```python
from build123d import *

# Parameters (mm, degrees)
IZIM1_R                     = 1.65
Y_KSEKLIK_EKSTR_ZYON1_DEPTH = 2.5
RADYUS1_RADIUS              = 3.5
RADYUS1_LENGTH              = 2.5
RADYUS3_R                   = 2
RADYUS4_R                   = 1.5
KES_EKSTR_ZYON1_DEPTH       = 52.79285665


with BuildPart() as part:
    # Çizim1 → Yükseklik-Ekstrüzyon1 (new body)
    with BuildSketch(Plane(origin=(0, 0, 0), x_dir=(0, 0, -1), z_dir=(1, 0, 0))):
        with BuildLine():
            Line((0, 0), (0, 26.5))
            ThreePointArc((0, 26.5), (-0.439339828, 27.560660172), (-1.5, 28))
            Line((-1.5, 28), (-35, 28))
            Line((-35, 28), (-35, 7))
            Line((-35, 7), (-43.5, 7))
            Line((-43.5, 7), (-43.5, 0))
            Line((-43.5, 0), (0, 0))
        make_face()
        with Locations((-17.5, 23.3)):
            Circle(IZIM1_R, mode=Mode.SUBTRACT)
        with Locations((-17.5, 4.7)):
            Circle(IZIM1_R, mode=Mode.SUBTRACT)
        with Locations((-30.9, 6.2)):
            Circle(IZIM1_R, mode=Mode.SUBTRACT)
        with Locations((-30.9, 21.8)):
            Circle(IZIM1_R, mode=Mode.SUBTRACT)
        with Locations((-4.1, 6.2)):
            Circle(IZIM1_R, mode=Mode.SUBTRACT)
        with Locations((-4.1, 21.8)):
            Circle(IZIM1_R, mode=Mode.SUBTRACT)
        with Locations((-40, 3.5)):
            Circle(IZIM1_R, mode=Mode.SUBTRACT)
    extrude(amount=Y_KSEKLIK_EKSTR_ZYON1_DEPTH)

    # Radyus1: full round fillet: the end face becomes a half cylinder, R = half its width
    radyus1_face = Plane((1.25, 3.5, 43.5), x_dir=(1, 0, 0), z_dir=(0, 0, 1))  # on the end face: x along it, z out of the body
    radyus1_slab = radyus1_face.offset(-RADYUS1_RADIUS / 2) * Box(RADYUS1_LENGTH, 2 * RADYUS1_RADIUS, RADYUS1_RADIUS, mode=Mode.PRIVATE)  # the body's end, R deep
    radyus1_round = Plane((1.25, 3.5, 40), x_dir=(0, 0, 1), z_dir=(1, 0, 0)) * Cylinder(RADYUS1_RADIUS, RADYUS1_LENGTH, mode=Mode.PRIVATE)  # its axis R under the face
    add(radyus1_slab - radyus1_round, mode=Mode.SUBTRACT)

    # Radyus3
    radyus3_edges = [part.edges().sort_by_distance(p)[0] for p in [
        (1.25, 7, 35),
    ]]
    fillet(radyus3_edges, radius=RADYUS3_R)

    # Radyus4
    radyus4_edges = [part.edges().sort_by_distance(p)[0] for p in [
        (1.25, 28, 35),
    ]]
    fillet(radyus4_edges, radius=RADYUS4_R)

    # Çizim2 → Kes-Ekstrüzyon1 (cut, through all)
    with BuildSketch(Plane(origin=(2.5, 0, 0), x_dir=(0, 0, -1), z_dir=(1, 0, 0))):
        with BuildLine():
            Line((-33.5, 16.8), (-33.5, 11.8))
            ThreePointArc((-33.5, 11.8), (-33.060660172, 10.739339828), (-32, 10.3))
            Line((-32, 10.3), (-28, 10.3))
            ThreePointArc((-28, 10.3), (-26.648045146, 11.150216904), (-26.828696786, 12.737042571))
            Line((-26.828696786, 12.737042571), (-30.828696786, 17.737042571))
            ThreePointArc((-30.828696786, 17.737042571), (-32.496510412, 18.215442479), (-33.5, 16.8))
        make_face()
        with BuildLine():
            Line((-25, 18.3), (-21, 18.3))
            ThreePointArc((-21, 18.3), (-19.939339828, 17.860660172), (-19.5, 16.8))
            Line((-19.5, 16.8), (-19.5, 11.8))
            ThreePointArc((-19.5, 11.8), (-20.503489588, 10.384557521), (-22.171303214, 10.862957429))
            Line((-22.171303214, 10.862957429), (-26.171303214, 15.862957429))
            ThreePointArc((-26.171303214, 15.862957429), (-26.351954854, 17.449783096), (-25, 18.3))
        make_face()
        with BuildLine():
            Line((-12.828696786, 10.862957429), (-8.828696786, 15.862957429))
            ThreePointArc((-8.828696786, 15.862957429), (-8.648045146, 17.449783096), (-10, 18.3))
            Line((-10, 18.3), (-14, 18.3))
            ThreePointArc((-14, 18.3), (-15.060660172, 17.860660172), (-15.5, 16.8))
            Line((-15.5, 16.8), (-15.5, 11.8))
            ThreePointArc((-15.5, 11.8), (-14.496510412, 10.384557521), (-12.828696786, 10.862957429))
        make_face()
        with BuildLine():
            Line((-8.171303214, 12.737042571), (-4.171303214, 17.737042571))
            ThreePointArc((-4.171303214, 17.737042571), (-2.503489588, 18.215442479), (-1.5, 16.8))
            Line((-1.5, 16.8), (-1.5, 11.8))
            ThreePointArc((-1.5, 11.8), (-1.939339828, 10.739339828), (-3, 10.3))
            Line((-3, 10.3), (-7, 10.3))
            ThreePointArc((-7, 10.3), (-8.351954854, 11.150216904), (-8.171303214, 12.737042571))
        make_face()
    extrude(amount=-KES_EKSTR_ZYON1_DEPTH, mode=Mode.SUBTRACT)


solid = part.part
```
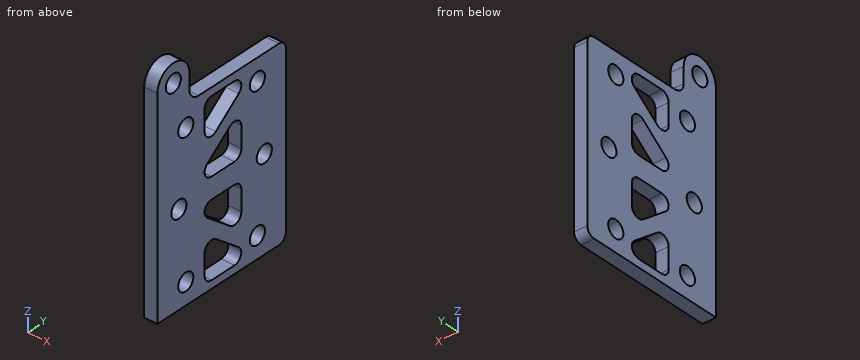
Design review of the part built by this model. Coordinates are the model's own, in mm. Coordinates: 2 decimals unless noted, no trailing zeros. Order: outer loops, then holes, each group sorted by start corner. A loop starts at its lowest first (then second) coordinate and runs counter-clockwise, first axis right, second up. Notation, with made-up numbers: M 27.25,79 L 32.25,79 A22 ccw 32.25,108 Z; hole C 43,41.5 d9. An arc over 180 degrees is marked long. Answer as a JSON object with one key per item and string values. Group by question number.
1) Add section A-A, the plane z = 17.5. Write out the cut boundary in (x, y), then the cut area to 3 significant figures.
2) Wall thickness on L1, parallel to Y at x = 1.7, z = 17.5; L2, parallel to Z at x = 0.3, y = 4.5; L3, parallel to Y at x = 0.75, z = 30.9: over which ranges is each line inside the solid? List them lowest first.
3) Add section C-C, the plane y = 19.25. Write out the cut boundary in (x, z).
4) For pin 1 (0.8 mm diameter, centred on x = 1, z = 13, fed in from -Y); pin 2 (0.8 mm diameter, centred on x = 1, y = 15, fed in from +Z); pin 3 (2.5 mm diameter, centred on y = 21.8, z = 4.1, fed in from +X), all flat-tipped, find the tip position at first contact; note any pin that passes through.
5) Add section D-D, the plane z = 25.5. Write out the cut boundary in (x, y).
6) Add section B-B, the plane x = 1.95. Count the separate pieces of the cut face and the enclosed holes in it, then the cut area to 3 significant figures.
Computed values:
{
 "1": {"outline": "M 0,0 L 2.5,0 L 2.5,3.05 L 0,3.05 Z; M 0,6.35 L 2.5,6.35 L 2.5,21.65 L 0,21.65 Z; M 0,24.95 L 2.5,24.95 L 2.5,28 L 0,28 Z", "area": "53.5 mm^2"},
 "2": {"L1": "y = 0 to 3.05, 6.35 to 21.65, 24.95 to 28", "L2": "z = 0 to 15.86, 19.14 to 38.69, 41.31 to 43.35", "L3": "y = 0 to 4.55, 7.85 to 10.3, 17.82 to 20.15, 23.45 to 28"},
 "3": {"outline": "M 0,0 L 2.5,0 L 2.5,35 L 0,35 Z"},
 "4": {"pin 1": "stops at y = 0", "pin 2": "stops at z = 35", "pin 3": "passes through"},
 "5": {"outline": "M 0,0 L 2.5,0 L 2.5,15.02 L 0,15.02 Z; M 0,18.21 L 2.5,18.21 L 2.5,28 L 0,28 Z"},
 "6": {"separate pieces": "1", "enclosed holes": "11", "area": "814 mm^2"}
}
